Autodesk Inventor part; units mm, degrees
ref_plane "Work Plane1" through (-13.8343, -45.838, 7.888) normal (0, 0, -1) x (0, 1, 0)
ref_plane "YZ Plane" through (0, 0, 0) normal (1, 0, 0) x (0, 1, 0)
ref_plane "XZ Plane" through (0, 0, 0) normal (0, 1, 0) x (-1, 0, 0)
sketch "Sketch1" plane through (0, 0, 0) normal (0, 0, 1) x (1, 0, 0)
  arc A0 (-3.52, 5.9525) -> (-4.52, 4.9525) centre (-3.52, 4.9525) ccw
  line L0 (-4.52, -4.8041) -> (-4.52, 4.9525)
  arc A1 (-4.52, -4.8041) -> (-3.52, -5.8041) centre (-3.52, -4.8041) ccw
  line L1 (-2.52, -5.8041) -> (-3.52, -5.8041)
  arc A2 (-2.52, -5.8041) -> (-1.52, -4.8041) centre (-2.52, -4.8041) ccw
  line L2 (-1.52, 0.9525) -> (-1.52, -4.8041)
  line L3 (1.52, 0.9525) -> (-1.52, 0.9525)
  line L4 (1.52, -4.8041) -> (1.52, 0.9525)
  arc A3 (1.52, -4.8041) -> (2.52, -5.8041) centre (2.52, -4.8041) ccw
  line L5 (3.52, -5.8041) -> (2.52, -5.8041)
  arc A4 (3.52, -5.8041) -> (4.52, -4.8041) centre (3.52, -4.8041) ccw
  line L6 (4.52, 4.9525) -> (4.52, -4.8041)
  arc A5 (4.52, 4.9525) -> (3.52, 5.9525) centre (3.52, 4.9525) ccw
  line L7 (-3.52, 5.9525) -> (3.52, 5.9525)
  arc A6 (2.52, -28.2909) -> (1.52, -29.2909) centre (2.52, -29.2909) ccw
  line L8 (1.52, -35.0475) -> (1.52, -29.2909)
  line L9 (-1.52, -35.0475) -> (1.52, -35.0475)
  line L10 (-1.52, -29.2909) -> (-1.52, -35.0475)
  arc A7 (-1.52, -29.2909) -> (-2.52, -28.2909) centre (-2.52, -29.2909) ccw
  line L11 (-3.52, -28.2909) -> (-2.52, -28.2909)
  arc A8 (-3.52, -28.2909) -> (-4.52, -29.2909) centre (-3.52, -29.2909) ccw
  line L12 (-4.52, -39.0475) -> (-4.52, -29.2909)
  arc A9 (-4.52, -39.0475) -> (-3.52, -40.0475) centre (-3.52, -39.0475) ccw
  line L13 (3.52, -40.0475) -> (-3.52, -40.0475)
  arc A10 (3.52, -40.0475) -> (4.52, -39.0475) centre (3.52, -39.0475) ccw
  line L14 (4.52, -29.2909) -> (4.52, -39.0475)
  arc A11 (4.52, -29.2909) -> (3.52, -28.2909) centre (3.52, -29.2909) ccw
  line L15 (2.52, -28.2909) -> (3.52, -28.2909)
  point P0 (0, 0)
extrude "Extrusion1" add sketch "Sketch1" along normal blind 5
sketch "Sketch2" plane through (0, 0, 5) normal (0, 0, 1) x (1, 0, 0)
  arc A0 (-3.52, 5.9525) -> (-4.52, 4.9525) centre (-3.52, 4.9525) ccw
  line L0 (-4.52, 4.9525) -> (-4.52, -4.8041)
  arc A1 (-4.52, -4.8041) -> (-3.52, -5.8041) centre (-3.52, -4.8041) ccw
  line L1 (-3.52, -5.8041) -> (-2.52, -5.8041)
  arc A2 (-2.52, -5.8041) -> (-1.52, -4.8041) centre (-2.52, -4.8041) ccw
  line L2 (-1.52, -4.8041) -> (-1.52, 0.9525)
  line L3 (-1.52, 0.9525) -> (1.52, 0.9525)
  line L4 (1.52, 0.9525) -> (1.52, -4.8041)
  arc A3 (1.52, -4.8041) -> (2.52, -5.8041) centre (2.52, -4.8041) ccw
  line L5 (2.52, -5.8041) -> (3.52, -5.8041)
  arc A4 (3.52, -5.8041) -> (4.52, -4.8041) centre (3.52, -4.8041) ccw
  line L6 (4.52, -4.8041) -> (4.52, 4.9525)
  arc A5 (4.52, 4.9525) -> (3.52, 5.9525) centre (3.52, 4.9525) ccw
  line L7 (3.52, 5.9525) -> (-3.52, 5.9525)
  arc A6 (2.52, -28.2909) -> (1.52, -29.2909) centre (2.52, -29.2909) ccw
  line L8 (1.52, -29.2909) -> (1.52, -35.0475)
  line L9 (1.52, -35.0475) -> (-1.52, -35.0475)
  line L10 (-1.52, -35.0475) -> (-1.52, -29.2909)
  arc A7 (-1.52, -29.2909) -> (-2.52, -28.2909) centre (-2.52, -29.2909) ccw
  line L11 (-2.52, -28.2909) -> (-3.52, -28.2909)
  arc A8 (-3.52, -28.2909) -> (-4.52, -29.2909) centre (-3.52, -29.2909) ccw
  line L12 (-4.52, -29.2909) -> (-4.52, -39.0475)
  arc A9 (-4.52, -39.0475) -> (-3.52, -40.0475) centre (-3.52, -39.0475) ccw
  line L13 (-3.52, -40.0475) -> (3.52, -40.0475)
  arc A10 (3.52, -40.0475) -> (4.52, -39.0475) centre (3.52, -39.0475) ccw
  line L14 (4.52, -39.0475) -> (4.52, -29.2909)
  arc A11 (4.52, -29.2909) -> (3.52, -28.2909) centre (3.52, -29.2909) ccw
  line L15 (3.52, -28.2909) -> (2.52, -28.2909)
  line L16 (-4.52, -4.8041) -> (4.52, -4.8041)
  line L17 (4.52, -4.8041) -> (4.52, -29.2909)
  line L18 (4.52, -29.2909) -> (-4.52, -29.2909)
  line L19 (-4.52, -29.2909) -> (-4.52, -4.8041)
  line L20 (-1.52, -35.0475) -> (1.52, -35.0475)
  line L21 (1.52, -35.0475) -> (1.52, 0.9525)
  line L22 (1.52, 0.9525) -> (-1.52, 0.9525)
  line L23 (-1.52, 0.9525) -> (-1.52, -35.0475)
  point P0 (0, 0)
ref_plane "Work Plane1" through (-13.8343, -45.838, 7.888) normal (0, 0, -1) x (0, 1, 0)
extrude "Extrusion2" add sketch "Sketch2" along normal up to surface (2.888 mm away)
sketch "Sketch3" plane through (-3.52, 5.9525, 7.888) normal (0, 0, 1) x (1, 0, 0)
  arc A0 (6.04, -34.2434) -> (5.04, -35.2434) centre (6.04, -35.2434) ccw
  line L0 (5.04, -41) -> (5.04, -35.2434)
  line L1 (2, -41) -> (5.04, -41)
  line L2 (2, -35.2434) -> (2, -41)
  arc A1 (2, -35.2434) -> (1, -34.2434) centre (1, -35.2434) ccw
  line L3 (0, -34.2434) -> (1, -34.2434)
  arc A2 (0, -34.2434) -> (-1, -35.2434) centre (0, -35.2434) ccw
  line L4 (-1, -45) -> (-1, -35.2434)
  arc A3 (-1, -45) -> (0, -46) centre (0, -45) ccw
  line L5 (7.04, -46) -> (0, -46)
  arc A4 (7.04, -46) -> (8.04, -45) centre (7.04, -45) ccw
  line L6 (8.04, -35.2434) -> (8.04, -45)
  arc A5 (8.04, -35.2434) -> (7.04, -34.2434) centre (7.04, -35.2434) ccw
  line L7 (6.04, -34.2434) -> (7.04, -34.2434)
  arc A6 (0, 0) -> (-1, -1) centre (0, -1) ccw
  line L8 (-1, -10.7566) -> (-1, -1)
  arc A7 (-1, -10.7566) -> (0, -11.7566) centre (0, -10.7566) ccw
  line L9 (1, -11.7566) -> (0, -11.7566)
  arc A8 (1, -11.7566) -> (2, -10.7566) centre (1, -10.7566) ccw
  line L10 (2, -5) -> (2, -10.7566)
  line L11 (5.04, -5) -> (2, -5)
  line L12 (5.04, -10.7566) -> (5.04, -5)
  arc A9 (5.04, -10.7566) -> (6.04, -11.7566) centre (6.04, -10.7566) ccw
  line L13 (7.04, -11.7566) -> (6.04, -11.7566)
  arc A10 (7.04, -11.7566) -> (8.04, -10.7566) centre (7.04, -10.7566) ccw
  line L14 (8.04, -1) -> (8.04, -10.7566)
  arc A11 (8.04, -1) -> (7.04, 0) centre (7.04, -1) ccw
  line L15 (0, 0) -> (7.04, 0)
  line L16 (0, -46) -> (7.04, -46)
  line L17 (3.52, -46) -> (3.52, -41)
  line L18 (2, -41) -> (5.04, -41)
  circle A12 centre (3.52, -43.5) radius 1.375
  circle A13 centre (3.52, -43.5) radius 1.375
  line L19 (-1, -1) -> (-1, -45)
  line L20 (-1, -23) -> (-5.6453, -23)
  arc A14 (5.04, -10.7566) -> (6.04, -11.7566) centre (6.04, -10.7566) ccw
  line L21 (5.04, -5) -> (5.04, -10.7566)
  line L22 (2, -5) -> (5.04, -5)
  line L23 (2, -10.7566) -> (2, -5)
  arc A15 (1, -11.7566) -> (2, -10.7566) centre (1, -10.7566) ccw
  line L24 (0, -11.7566) -> (1, -11.7566)
  arc A16 (-1, -10.7566) -> (0, -11.7566) centre (0, -10.7566) ccw
  line L25 (-1, -1) -> (-1, -10.7566)
  arc A17 (0, 0) -> (-1, -1) centre (0, -1) ccw
  line L26 (7.04, 0) -> (0, 0)
  arc A18 (8.04, -1) -> (7.04, 0) centre (7.04, -1) ccw
  line L27 (8.04, -10.7566) -> (8.04, -1)
  arc A19 (7.04, -11.7566) -> (8.04, -10.7566) centre (7.04, -10.7566) ccw
  line L28 (6.04, -11.7566) -> (7.04, -11.7566)
  line L29 (0, 0) -> (7.04, 0)
  line L30 (3.52, 0) -> (3.52, -5)
  line L31 (2, -5) -> (5.04, -5)
  circle A20 centre (3.52, -2.5) radius 1.375
  circle A21 centre (3.52, -2.5) radius 1.375
  line L32 (-1, -45) -> (-1, -1)
  point P0 (3.52, -5.9525)
  dimension "d5" = 2.75
  dimension "d6" = 2.75
extrude "Extrusion3" cut sketch "Sketch3" against normal blind 100 contours A12 L17 | L17 A12 | A20 L30 | L30 A20
properties part number "SyringeServoClamp"
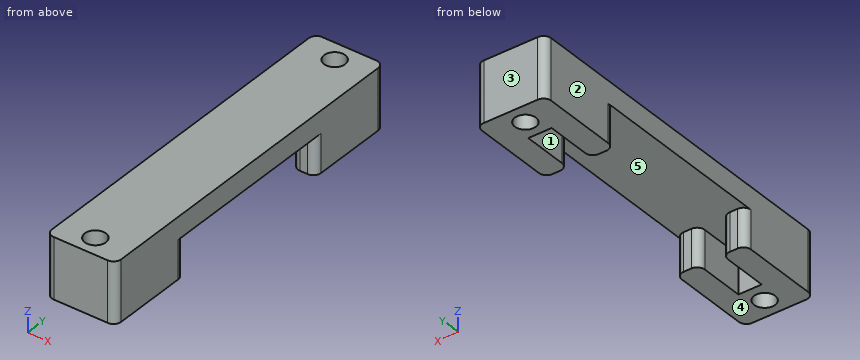
Read the model definition and answer for the solid it produces. Units are mm, in the model's axes. Face numbers are marked on the shaded views. A direction names the side the tool comes from. Give positions to 0.01 mm unless a question says otherwise; leave off trailing zeros. Write each loop counter-clockwise with the first axis right and the second up, starting at its lowest first coordinate (ties: lowest second). Pieces come first, ordered by that corner, then holes. Notation, with made-up numbers: (-35.5, 37) - (-13.5, 37) arc R12 cw to (-13.5, 50) - close; hole circle Ø1 at (14.5, 17). An arc over 180 degrees is marked (long way). Write item = value, one per line. Start each with the question number.
Item 1: Find section B-B (z = 6.25). State how many separate pieces and enclosed holes the cut face has, then the cut area to 3 significant figures.
Item 2: Find section C-C (y = 0). Give the vertices of the cut face in (x, z).
Item 3: Find section A-A (x = 0). Give the vertices of the cut face in (y, z).
Item 4: Find the intervals of material crossed by probe 1 along Y at (x, z) = (0, 4); probe 2 along Y at (x, z) = (0, 6.25); probe 3 along Z at (x, y) = (2, -13.5), in increasing order. Write a range as [from, to].
Item 5: Each of these flat-tipped pins is pushed along its axis until it touches: P1, Ø4.5, axis at x = 2, y = -19.5, coming from the -Z side; P2, Ø4, axis at y = -21.5, z = 2.5, coming from the +X side. Where does it stop, or does it pass through?
Item 6: A tool of negligible diameter and unlimited length cuts with its end or side. For the marked faces 4 and 5, from which of +Z, -Z, +X, -X, +Y, -Y can it reach the whole face along a straight path? Write none if from no direction.
Item 7: The mould has two halves that part along Y. Classify the marked faces 1, 2 and 3: +Y half, -Y half, draft (parallel to the pull), parting line (faces both ways), or undercut.
Response:
q1.separate_pieces = 1
q1.enclosed_holes = 2
q1.area = 403 mm²
q2.outline = (-4.52, 0) - (-1.52, 0) - (-1.52, 5) - (1.52, 5) - (1.52, 0) - (4.52, 0) - (4.52, 7.89) - (-4.52, 7.89) - close
q3.outline = (-40.05, 0) - (-38.92, 0) - (-38.92, 7.89) - (-40.05, 7.89) - close; (-36.17, 0) - (-35.05, 0) - (-35.05, 5) - (0.95, 5) - (0.95, 0) - (2.08, 0) - (2.08, 7.89) - (-36.17, 7.89) - close; (4.83, 0) - (5.95, 0) - (5.95, 7.89) - (4.83, 7.89) - close
q4.probe_1 = [-40.05, -38.92], [-36.17, -35.05], [0.95, 2.08], [4.83, 5.95]
q4.probe_2 = [-40.05, -38.92], [-36.17, 2.08], [4.83, 5.95]
q4.probe_3 = [5, 7.89]
q5.P1 = 5
q5.P2 = through
q6.face_4 = -Z, +X, -X, +Y, -Y
q6.face_5 = -Z
q7.face_1 = undercut
q7.face_2 = draft
q7.face_3 = +Y half
